Geometry: final body of the model. Coordinates: model frame, mm. A direction names the side the tool comes from. Coordinates: 2 decimals unless noted, no trailing zeros. Write each loop counter-clockwise with the first axis right and the second up, starting at its lowest first coordinate (ties: lowest second). Pieces come first, ordered by that corner, then holes. Notation, with made-up numbers: (84, 60.25) - (125, 60.25) arc R22 cw to (125, 94.25) - close; hole circle Ø4 at (72, 15.25). An arc over 180 degrees is marked (long way). Put each result on its own line as item: value.
```python
from build123d import *

# Parameters (mm, degrees)
F0_W     = 3
F0_H     = 10
F0_H_2   = 5
F1_DEPTH = 5
F2_START = -5
F2_DEPTH = 5
F3_DEPTH = 5


with BuildPart() as f1:
    # F0 (on Top) → F1 (new body)
    with BuildSketch(Plane.XY):
        with Locations((3.5, 7)):
            Rectangle(F0_W, F0_H)
        with BuildLine():
            Line((10.9485099174, 12), (5, 12))
            Line((5, 12), (5, 2))
            Line((5, 2), (11.9710084021, 2))
            ThreePointArc((11.9710084021, 2), (11.6421053306, 7.0186448683), (10.9485099174, 12))
        make_face()
        Polygon((5, 2), (2, 2), (2, -2), (5, -2), (5, 0), align=None)
        with BuildLine():
            Line((11.9710084021, 2), (5, 2))
            Line((5, 2), (5, 0))
            Line((5, 0), (5, -2))
            Line((5, -2), (11.9710084021, -2))
            ThreePointArc((11.9710084021, -2), (11.9927517198, -1.0001050586), (12, 0))
            ThreePointArc((12, 0), (11.9927517198, 1.0001050586), (11.9710084021, 2))
        make_face()
        with Locations((3.5, -4.5)):
            Rectangle(F0_W, F0_H_2)
        with BuildLine():
            Line((11.9710084021, -2), (5, -2))
            Line((5, -2), (5, -7))
            Line((5, -7), (11.6440092069, -7))
            ThreePointArc((11.6440092069, -7), (11.8529103806, -4.5029692558), (11.9710084021, -2))
        make_face()
    extrude(amount=-F1_DEPTH)



with BuildPart() as f1b:
    # F0 (on Top) → F1, piece 2 (new body)
    with BuildSketch(Plane.XY):
        with Locations((-3.5, 7)):
            Rectangle(F0_W, F0_H)
        with BuildLine():
            Line((-5, 2), (-5, 12))
            Line((-5, 12), (-10.9485099174, 12))
            ThreePointArc((-10.9485099174, 12), (-11.6421053306, 7.0186448683), (-11.9710084021, 2))
            Line((-11.9710084021, 2), (-5, 2))
        make_face()
        Polygon((-2, -2), (-2, 2), (-5, 2), (-5, 0), (-5, -2), align=None)
        with BuildLine():
            Line((-5, 0), (-5, 2))
            Line((-5, 2), (-11.9710084021, 2))
            ThreePointArc((-11.9710084021, 2), (-11.9927517198, 1.0001050586), (-12, 0))
            ThreePointArc((-12, 0), (-11.9927517198, -1.0001050586), (-11.9710084021, -2))
            Line((-11.9710084021, -2), (-5, -2))
            Line((-5, -2), (-5, 0))
        make_face()
        with Locations((-3.5, -4.5)):
            Rectangle(F0_W, F0_H_2)
        with BuildLine():
            Line((-5, -7), (-5, -2))
            Line((-5, -2), (-11.9710084021, -2))
            ThreePointArc((-11.9710084021, -2), (-11.8529103806, -4.5029692558), (-11.6440092069, -7))
            Line((-11.6440092069, -7), (-5, -7))
        make_face()
    extrude(amount=-F1_DEPTH)


with BuildPart() as f1_1:
    add(f1.part)

    add(f1b.part)  # F2 merges F1b
    # F0 (on Top) → F2 (join)
    with BuildSketch(Plane.XY.offset(F2_START)):
        Polygon((2, -2), (2, 2), (0, 2), (-2, 2), (-2, -2), (0, -2), align=None)
        Polygon((5, 2), (2, 2), (2, -2), (5, -2), (5, 0), align=None)
        Polygon((-2, -2), (-2, 2), (-5, 2), (-5, 0), (-5, -2), align=None)
        with BuildLine():
            Line((11.9710084021, 2), (5, 2))
            Line((5, 2), (5, 0))
            Line((5, 0), (5, -2))
            Line((5, -2), (11.9710084021, -2))
            ThreePointArc((11.9710084021, -2), (11.9927517198, -1.0001050586), (12, 0))
            ThreePointArc((12, 0), (11.9927517198, 1.0001050586), (11.9710084021, 2))
        make_face()
        with BuildLine():
            Line((-5, 0), (-5, 2))
            Line((-5, 2), (-11.9710084021, 2))
            ThreePointArc((-11.9710084021, 2), (-11.9927517198, 1.0001050586), (-12, 0))
            ThreePointArc((-12, 0), (-11.9927517198, -1.0001050586), (-11.9710084021, -2))
            Line((-11.9710084021, -2), (-5, -2))
            Line((-5, -2), (-5, 0))
        make_face()
    extrude(amount=-F2_DEPTH)

    # F0 (on Top) → F3 (join)
    with BuildSketch(Plane.XY):
        with BuildLine():
            ThreePointArc((-2, 57), (0, 59), (2, 57))
            Line((2, 57), (2, 12))
            Line((2, 12), (5, 12))
            Line((5, 12), (5, 57))
            ThreePointArc((5, 57), (0, 62), (-5, 57))
            Line((-5, 57), (-5, 12))
            Line((-5, 12), (-2, 12))
            Line((-2, 12), (-2, 57))
        make_face()
        with Locations((3.5, 7)):
            Rectangle(F0_W, F0_H)
        with Locations((-3.5, 7)):
            Rectangle(F0_W, F0_H)
        Polygon((5, 2), (2, 2), (2, -2), (5, -2), (5, 0), align=None)
        Polygon((-2, -2), (-2, 2), (-5, 2), (-5, 0), (-5, -2), align=None)
        with Locations((3.5, -4.5)):
            Rectangle(F0_W, F0_H_2)
        with Locations((-3.5, -4.5)):
            Rectangle(F0_W, F0_H_2)
        with BuildLine():
            Line((5, -7), (2, -7))
            Line((2, -7), (2, -57))
            ThreePointArc((2, -57), (0, -59), (-2, -57))
            Line((-2, -57), (-2, -7))
            Line((-2, -7), (-5, -7))
            Line((-5, -7), (-5, -57))
            ThreePointArc((-5, -57), (0, -62), (5, -57))
            Line((5, -57), (5, -7))
        make_face()
    extrude(amount=F3_DEPTH)


solid = f1_1.part
```
1. Section query C-C (y = 35.5). Return loops of the section in (x, z).
Answer below:
outline: (-5, 0) - (-2, 0) - (-2, 5) - (-5, 5) - close; (2, 0) - (5, 0) - (5, 5) - (2, 5) - close
2. Set-up query: faces 4 (the flat face through (8, 3, 0)), 5 (the flat face through (2, 1, 2)), 6 (the flat face through (-7, 7, -5)). Return all of +Z, -Z, +X, -X, +Y, -Y with unobstructed straight access to the full face (end or side cutting, diameter ignored); none if empty.
Answer below:
face 4: +Z, +X, +Y, -Y
face 5: +Z
face 6: -Z, +X, -X, +Y
3. Ray query, probe 1 along X at (y, z) = (-55, 3.75); probe 2 along Y at (x, z) = (4, -2.5); probe 3 along Z at (x, y) = (-7.75, -0.5). Return the intervals inside material, ascending. Write a range as from..to.
Answer below:
probe 1: x = -5..-2, 2..5
probe 2: y = -7..12
probe 3: z = -10..0
4. Pin query (flat end, axial travel): pin 1 Ø7.5 at (x, y) = (-9, 0) entering from +Z; pin 2 Ø8 at (y, z) = (24.5, -2.5) entering from +X; pin 3 Ø2.5 at (x, z) = (-8, -3) entering from -Y. Return the tip coordinate at first contact, or that it passes through.
Answer below:
pin 1: stops at z = 0
pin 2: stops at x = 5
pin 3: stops at y = -7
5. Section query B-B (z = -3.75). Return loops of the section in (x, y).
Answer below:
outline: (-11.64, -7) - (-2, -7) - (-2, 12) - (-10.95, 12) arc R69 ccw to start; (2, -7) - (11.64, -7) arc R69 ccw to (10.95, 12) - (2, 12) - close
6. Section query A-A (x = 0). Return loops of the section in (y, z), then the cut area to 3 significant figures.
Answer below:
outline: (-62, 0) - (-59, 0) - (-59, 5) - (-62, 5) - close; (-2, -10) - (2, -10) - (2, -5) - (-2, -5) - close; (59, 0) - (62, 0) - (62, 5) - (59, 5) - close
area: 50.0 mm²
7. Mould query, pull axis Y, two halves, no side actions, for faces 1 (the flat face through (5, -1, 2)), 2 (the flat face through (7, -7, -2)), 3 (the flat face through (-2, -1, 2)). Classes: +Y half, -Y half, draft (parallel to the pull), parting line (faces both ways), or undercut.
Answer below:
face 1: draft
face 2: -Y half
face 3: undercut
